The listing builds one solid part. Answer for the finished solid, in the listing's coordinates (mm). Face numbers are marked on the shaded views. A direction names the side the tool comes from. Coordinates: 2 decimals unless noted, no trailing zeros. Loops run counter-clockwise (first coordinate to the right, second up) from the corner with the lowest first, then second, coordinate; pieces in that order, holes last. Notation, with made-up numbers: M 87.25,51 L 98.25,51 A24 ccw 98.25,88 Z; hole C 67.25,8.25 d9. An arc over 180 degrees is marked long. Answer in a Markdown table with one row per item. Add a question column.
from build123d import *

# Parameters (mm, degrees)
F1_DEPTH = 48.26
F3_DEPTH = 18.288
F5_DEPTH = 25.4


with BuildPart() as f1:
    # F0 (on Top) → F1 (new body)
    with BuildSketch(Plane.XY):
        Polygon((-28.448, 0), (0, 0), (0, 30.48), (0, 60.96), (-28.448, 60.96), (-28.448, 48.26), (-18.288, 48.26), (-18.288, 43.18), (-18.288, 30.48), (-18.288, 17.78), (-18.288, 12.7), (-28.448, 12.7), align=None)
    extrude(amount=F1_DEPTH)

    # F2 (on face) → F3 (cut, through all)
    with BuildSketch(Plane.YZ):
        Polygon((17.78, 38.1), (30.48, 38.1), (43.18, 38.1), (43.18, 48.26), (17.78, 48.26), align=None)
    extrude(amount=-F3_DEPTH, mode=Mode.SUBTRACT)

    # F4 (on face) → F5 (join)
    with BuildSketch(Plane.XY.offset(48.26)):
        Polygon((0, 48.26), (0, 30.48), (0, 12.7), (60.198, 12.7), (90.932, 30.48), (60.198, 48.26), align=None)
    extrude(amount=-F5_DEPTH)


solid = f1.part
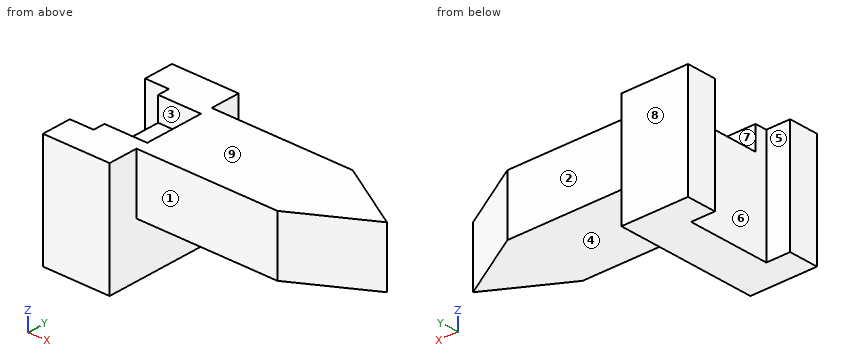
(1) For the marked faces 1, 2, 3, 4 and 5, determine the directions among +Z, -Z, +X, -X, +Y, -Y from which every point of the face is accessible in a straight line to the end or side of a thin tool.
(2) The mould has two halves that part along Y. Classify the marked faces 6, 7, 8 and 9: released by +Y, released by -Y, zero draft, split by the parting line, or undercut.
(3) A cutting plane is placed at C-C (x = 22). Give the vertices of the cut face in (y, z).
(4) Straight lines are drawn through the part: line 1 (Y direction, x = -23, z = 3); line 2 (Z direction, x = 33, y = 15.5); line 3 (X direction, y = 51, z = 9.5). For each, find the intervals that lie inside material, in ascending order.
(5) A cutting plane is placed at B-B (y = 33.5). Give the vertices of the cut face in (x, z), plus the area to 3 significant figures.
(6) Each of these flat-tipped pins is pushed along its axis until it touches: pin 1 (9 mm diameter, centred on x = -11.5, y = 29.5, fed in from +Z); pin 2 (7.5 mm diameter, centred on x = 26.5, z = 34.5, fed in from -Y); pin 3 (1 mm diameter, centred on y = 17, z = 40, fed in from -X); pin 4 (3 mm diameter, centred on x = 52, z = 21, fed in from -Y). Where does it stop, or does it pass through?
(7) A cutting plane is placed at A-A (z = 8). Give the vertices of the cut face in (x, y), plus the area to 3 significant figures.
(8) A cutting plane is placed at D-D (z = 40). Give the vertices of the cut face in (x, y), plus the area to 3 significant figures.
Solved:
| question | item | result |
|---|---|---|
| 1 | face 1 | +Z, -Z, +X, -Y |
| 1 | face 2 | +Z, -Z, +X, +Y |
| 1 | face 3 | +Z, -X |
| 1 | face 4 | -Z, +X, +Y, -Y |
| 1 | face 5 | +Z, -Z, -X |
| 2 | face 6 | undercut |
| 2 | face 7 | undercut |
| 2 | face 8 | released by +Y |
| 2 | face 9 | zero draft |
| 3 | outline | M 12.7,22.86 L 48.26,22.86 L 48.26,48.26 L 12.7,48.26 Z |
| 4 | line 1 | y = 0 to 12.7, 48.26 to 60.96 |
| 4 | line 2 | z = 22.86 to 48.26 |
| 4 | line 3 | x = -28.45 to 0 |
| 5 | outline | M -18.29,0 L 0,0 L 0,22.86 L 85.71,22.86 L 85.71,48.26 L 0,48.26 L 0,38.1 L -18.29,38.1 Z |
| 5 | area | 2,870 mm² |
| 6 | pin 1 | stops at z = 38.1 |
| 6 | pin 2 | stops at y = 12.7 |
| 6 | pin 3 | stops at x = -18.29 |
| 6 | pin 4 | passes through |
| 7 | outline | M -28.45,0 L 0,0 L 0,60.96 L -28.45,60.96 L -28.45,48.26 L -18.29,48.26 L -18.29,12.7 L -28.45,12.7 Z |
| 7 | area | 1,370 mm² |
| 8 | outline | M -28.45,0 L 0,0 L 0,12.7 L 60.2,12.7 L 90.93,30.48 L 60.2,48.26 L 0,48.26 L 0,60.96 L -28.45,60.96 L -28.45,48.26 L -18.29,48.26 L -18.29,43.18 L 0,43.18 L 0,17.78 L -18.29,17.78 L -18.29,12.7 L -28.45,12.7 Z |
| 8 | area | 3,600 mm² |
